```python
from build123d import *

# Parameters (mm, degrees)
SKETCH1_R           = 1
BOSS_EXTRUDE1_DEPTH = 1.59


with BuildPart() as part:
    # Sketch1 → Boss-Extrude1 (new body)
    with BuildSketch(Plane(origin=(0, 0, 0), x_dir=(1, 0, 0), z_dir=(0, 1, 0))):
        with BuildLine():
            Line((-13.982567653, 7.132116323), (-22.861764958, 10.312114381))
            Line((-22.861764958, 10.312114381), (-24.21044114, 6.546337894))
            Line((-24.21044114, 6.546337894), (-16.738208265, 3.870230446))
            ThreePointArc((-16.738208265, 3.870230446), (-16.394250173, 3.660951485), (-16.160706095, 3.332984998))
            ThreePointArc((-16.160706095, 3.332984998), (-9.589384902, -2.894483489), (-0.541170736, -2.5887935))
            ThreePointArc((-0.541170736, -2.5887935), (-0.320283974, -2.517169363), (-0.088833144, -2.498421236))
            ThreePointArc((-0.088833144, -2.498421236), (2.19617582, 1.194492264), (-2.145600439, 1.283120709))
            ThreePointArc((-2.145600439, 1.283120709), (-2.359359709, 1.03174859), (-2.643290683, 0.863629079))
            ThreePointArc((-2.643290683, 0.863629079), (-8.831767295, 1.131940065), (-12.836874427, 5.857228461))
            ThreePointArc((-12.836874427, 5.857228461), (-13.266784954, 6.623123616), (-13.982567653, 7.132116323))
        make_face()
        Circle(SKETCH1_R, mode=Mode.SUBTRACT)
    extrude(amount=BOSS_EXTRUDE1_DEPTH)


solid = part.part
```
Check sheet for the modelled part. Datum: model origin and axes. Units: mm. Coordinates: 2 decimals unless noted, no trailing zeros. Loops run counter-clockwise (first coordinate to the right, second up) from the corner with the lowest first, then second, coordinate; pieces in that order, holes last.
1) Sectioned sample at D-D (z = -4.75). Record the boundary of the cut face in (x, y).
2) Release check for a two-part mould opening along X. For faces 1 (the face through (-18.36, 0.78, -8.7)), 2 (the face through (0, 1, 1)), 3 (the face through (-20.53, 0.78, -5.23)) record: released by +X, released by -X, zero draft, split by the parting line, or undercut.
3) Sectioned sample at C-C (z = -1.75). Record the boundary of the cut face in (x, y), and give its area (3 significant figures).
4) Sectioned sample at B-B (y = 1.05). Record the boundary of the cut face in (x, z).
5) Sectioned sample at A-A (z = 0.5). Record the boundary of the cut face in (x, y).
6) Material ranges on probe 1 along Z at (x, y) = (0, 0.45); probe 2 along X at (y, z) = (1.15, 0); probe 3 along Z at (x, y) = (-9.25, 1.15), recorded low to high.
Check sheet entries:
1. outline: (-19.19, 0) - (-12.41, 0) - (-12.41, 1.59) - (-19.19, 1.59) - close
2. face 1: released by +X
2. face 2: undercut
2. face 3: released by -X
3. outline: (-15.31, 0) - (-9.88, 0) - (-9.88, 1.59) - (-15.31, 1.59) - close; (-1.79, 0) - (1.79, 0) - (1.79, 1.59) - (-1.79, 1.59) - close
3. area: 14.3 mm2
4. outline: (-24.21, -6.55) - (-22.86, -10.31) - (-13.98, -7.13) arc R2.01 ccw to (-12.84, -5.86) arc R7.73 cw to (-2.64, -0.86) arc R1 cw to (-2.15, -1.28) arc R2.5 ccw (long way) to (-0.09, 2.5) arc R1 cw to (-0.54, 2.59) arc R11.73 ccw to (-16.16, -3.33) arc R1 cw to (-16.74, -3.87) - close; hole circle Ø2 at (0, 0)
5. outline: (-13.44, 0) - (-0.87, 0) - (-0.87, 1.59) - (-13.44, 1.59) - close; (0.87, 0) - (2.45, 0) - (2.45, 1.59) - (0.87, 1.59) - close
6. probe 1: z = -2.5 to -1, 1 to 2.5
6. probe 2: x = -13.94 to -1, 1 to 2.5
6. probe 3: z = -1.35 to 3.02
